```python
from build123d import *

# Parameters (mm, degrees)
CROQUIS1_W                   = 56
CROQUIS1_H                   = 82
CROQUIS1_W_2                 = 50
CROQUIS1_H_2                 = 76
EXTRUIR_L_MINA1_DEPTH        = 22
REDONDEO1_R                  = 4
REDONDEO2_R                  = 4
REDONDEO3_R                  = 4
REDONDEO4_R                  = 4
SALIENTE_EXTRUIR1_DEPTH      = 1
SALIENTE_EXTRUIR1_DEPTH_BACK = 1
REDONDEO5_R                  = 2
CROQUIS3_W                   = 6
CROQUIS3_H                   = 6.3
SALIENTE_EXTRUIR2_DEPTH      = 15.8
CROQUIS4_R                   = 0.75
CORTAR_EXTRUIR1_DEPTH        = 10
CROQUIS5_W                   = 10
CROQUIS5_H                   = 60.4
CORTAR_EXTRUIR2_DEPTH        = 10
CROQUIS6_W                   = 9
CROQUIS6_H                   = 67
CORTAR_EXTRUIR4_DEPTH        = 10
CROQUIS7_W                   = 3.2
CROQUIS7_H                   = 17
CORTAR_EXTRUIR5_DEPTH        = 10
CROQUIS8_W                   = 7.469429576
CROQUIS8_H                   = 3.762632311
SALIENTE_EXTRUIR3_DEPTH      = 22
CORTAR_EXTRUIR6_DEPTH        = 85
CROQUIS10_R                  = 1.25
CORTAR_EXTRUIR7_DEPTH        = 10
CROQUIS11_R                  = 1.1
CORTAR_EXTRUIR8_DEPTH        = 10


with BuildPart() as part:
    # Croquis1 → Extruir-Lámina1 (new body)
    with BuildSketch(Plane.XY):
        Rectangle(CROQUIS1_W, CROQUIS1_H)
        Rectangle(CROQUIS1_W_2, CROQUIS1_H_2, mode=Mode.SUBTRACT)
    extrude(amount=EXTRUIR_L_MINA1_DEPTH)

    # Redondeo1
    redondeo1_edges = [part.edges().sort_by_distance(p)[0] for p in [
        (-28, 41, 11),
    ]]
    fillet(redondeo1_edges, radius=REDONDEO1_R)

    # Redondeo2
    redondeo2_edges = [part.edges().sort_by_distance(p)[0] for p in [
        (28, 41, 11),
    ]]
    fillet(redondeo2_edges, radius=REDONDEO2_R)

    # Redondeo3
    redondeo3_edges = [part.edges().sort_by_distance(p)[0] for p in [
        (28, -41, 11),
    ]]
    fillet(redondeo3_edges, radius=REDONDEO3_R)

    # Redondeo4
    redondeo4_edges = [part.edges().sort_by_distance(p)[0] for p in [
        (-28, -41, 11),
    ]]
    fillet(redondeo4_edges, radius=REDONDEO4_R)

    # Croquis2 → Saliente-Extruir1 (add, two sides: drawn at the far end of the back side and taken through both)
    with BuildSketch(Plane.XY.offset(22).offset(-SALIENTE_EXTRUIR1_DEPTH_BACK)):
        with BuildLine():
            Line((-28, 37), (-28, -37))
            ThreePointArc((-28, -37), (-26.828427125, -39.828427125), (-24, -41))
            Line((-24, -41), (24, -41))
            ThreePointArc((24, -41), (26.828427125, -39.828427125), (28, -37))
            Line((28, -37), (28, 37))
            ThreePointArc((28, 37), (26.828427125, 39.828427125), (24, 41))
            Line((24, 41), (-24, 41))
            ThreePointArc((-24, 41), (-26.828427125, 39.828427125), (-28, 37))
        make_face()
    extrude(amount=SALIENTE_EXTRUIR1_DEPTH + SALIENTE_EXTRUIR1_DEPTH_BACK)

    # Redondeo5
    redondeo5_edges = [part.edges().sort_by_distance(p)[0] for p in [
        (-26.828427125, 39.828427125, 23),
        (-28, 0, 23),
        (-26.828427125, -39.828427125, 23),
        (0, -41, 23),
        (26.828427125, -39.828427125, 23),
        (28, 0, 23),
        (26.828427125, 39.828427125, 23),
        (0, 41, 23),
    ]]
    fillet(redondeo5_edges, radius=REDONDEO5_R)

    # Croquis3 → Saliente-Extruir2 (add)
    with BuildSketch(Plane(origin=(0, 0, 21), x_dir=(-1, 0, 0), z_dir=(0, 0, -1))):
        with Locations((-22, 34.85)):
            Rectangle(CROQUIS3_W, CROQUIS3_H)
        with Locations((-22, -34.85)):
            Rectangle(CROQUIS3_W, CROQUIS3_H)
        with Locations((22, 34.85)):
            Rectangle(CROQUIS3_W, CROQUIS3_H)
        with Locations((22, -34.85)):
            Rectangle(CROQUIS3_W, CROQUIS3_H)
    extrude(amount=SALIENTE_EXTRUIR2_DEPTH)

    # Croquis4 → Cortar-Extruir1 (cut)
    with BuildSketch(Plane(origin=(0, 0, 5.2), x_dir=(-1, 0, 0), z_dir=(0, 0, -1))):
        with Locations((-22, 34.5)):
            Circle(CROQUIS4_R)
        with Locations((22, 34.5)):
            Circle(CROQUIS4_R)
        with Locations((22, -34.5)):
            Circle(CROQUIS4_R)
        with Locations((-22, -34.5)):
            Circle(CROQUIS4_R)
    extrude(amount=-CORTAR_EXTRUIR1_DEPTH, mode=Mode.SUBTRACT)

    # Croquis5 → Cortar-Extruir2 (cut)
    with BuildSketch(Plane(origin=(0, 0, 21), x_dir=(-1, 0, 0), z_dir=(0, 0, -1))):
        with Locations((-20, 0)):
            Rectangle(CROQUIS5_W, CROQUIS5_H)
    extrude(amount=-CORTAR_EXTRUIR2_DEPTH, mode=Mode.SUBTRACT)

    # Croquis6 → Cortar-Extruir4 (cut)
    with BuildSketch(Plane(origin=(28, 0, 0), x_dir=(0, 0, -1), z_dir=(1, 0, 0))):
        with Locations((-11, 0)):
            Rectangle(CROQUIS6_W, CROQUIS6_H)
    extrude(amount=-CORTAR_EXTRUIR4_DEPTH, mode=Mode.SUBTRACT)

    # Croquis7 → Cortar-Extruir5 (cut)
    with BuildSketch(Plane(origin=(0, 0, 0), x_dir=(-1, 0, 0), z_dir=(0, 0, -1))):
        with Locations((25.4, -14.5)):
            Rectangle(CROQUIS7_W, CROQUIS7_H)
    extrude(amount=-CORTAR_EXTRUIR5_DEPTH, mode=Mode.SUBTRACT)

    # Croquis8 → Saliente-Extruir3 (add)
    with BuildSketch(Plane(origin=(0, 0, 0), x_dir=(-1, 0, 0), z_dir=(0, 0, -1))):
        with Locations((18.80938175, 42.881316156)):
            Rectangle(CROQUIS8_W, CROQUIS8_H)
        with Locations((-18.80938175, 42.881316156)):
            Rectangle(CROQUIS8_W, CROQUIS8_H)
        with Locations((-18.80938175, -42.881316156)):
            Rectangle(CROQUIS8_W, CROQUIS8_H)
        with Locations((18.80938175, -42.881316156)):
            Rectangle(CROQUIS8_W, CROQUIS8_H)
    extrude(amount=-SALIENTE_EXTRUIR3_DEPTH)

    # Croquis9 → Cortar-Extruir6 (cut)
    with BuildSketch(Plane(origin=(28, 0, 0), x_dir=(0, 0, -1), z_dir=(1, 0, 0))):
        Polygon((-21, 41), (0, 44.762632311), (0.10305202, 48.489025058), (-25.204298305, 46.436230698), (-22.314872849, 40.902663886), align=None)
        Polygon((-22.314872849, -40.902663886), (-21, -41), (0, -44.762632311), (0.10305202, -48.489025058), (-25.204298305, -46.436230698), align=None)
    extrude(amount=-CORTAR_EXTRUIR6_DEPTH, mode=Mode.SUBTRACT)

    # Croquis10 → Cortar-Extruir7 (cut)
    with BuildSketch(Plane(origin=(0, 0, 0), x_dir=(-1, 0, 0), z_dir=(0, 0, -1))):
        with Locations((-19, 41.25)):
            Circle(CROQUIS10_R)
        with Locations((19, 41.25)):
            Circle(CROQUIS10_R)
        with Locations((-19, -41.25)):
            Circle(CROQUIS10_R)
        with Locations((19, -41.25)):
            Circle(CROQUIS10_R)
    extrude(amount=-CORTAR_EXTRUIR7_DEPTH, mode=Mode.SUBTRACT)

    # Croquis11 → Cortar-Extruir8 (cut)
    with BuildSketch(Plane(origin=(0, 0, 5.2), x_dir=(-1, 0, 0), z_dir=(0, 0, -1))):
        with Locations((-22, 34.5)):
            Circle(CROQUIS11_R)
        with Locations((22, 34.5)):
            Circle(CROQUIS11_R)
        with Locations((22, -34.5)):
            Circle(CROQUIS11_R)
        with Locations((-22, -34.5)):
            Circle(CROQUIS11_R)
    extrude(amount=-CORTAR_EXTRUIR8_DEPTH, mode=Mode.SUBTRACT)


solid = part.part
```
Could you check a few things on this model? Use its own coordinates, in mm. A direction names the side the tool comes from. Round coordinates to 2 decimals unless told otherwise and drop trailing zeros. Loops run counter-clockwise (first coordinate to the right, second up) from the corner with the lowest first, then second, coordinate; pieces in that order, holes last. Notation, with made-up numbers: M 59,44 L 108,44 A23 ccw 108,78 Z; hole C 8,17 d11. An arc over 180 degrees is marked long. Write item = value, one per line.
1. I need wall thicknesses on probe 1 along Y at (x, z) = (11, 1.25); probe 2 along Y at (x, z) = (-22, 9.5); probe 3 along X at (y, z) = (24, 2). Which ranges of each line are inside material? Lowest first, please.
Results below:
probe_1 = -41 to -38, 38 to 41
probe_2 = -43.06 to -35.6, -33.4 to -31.7, 31.7 to 33.4, 35.6 to 43.06
probe_3 = -28 to -25, 25 to 28
2. Will these pins go through, and if not, where does the flat tip stop? P1, Ø1.1, axis at x = -22.5, y = -35, coming from the -Z side; P2, Ø1.6, axis at x = 23, z = 7.5, coming from the +Y side; P3, Ø1.9, axis at y = -43.5, z = 10.5, coming from the +X side.
Results below:
P1 = 5.2
P2 = 43.54
P3 = 22.54
3. I want a section at C-C, the plane z = 13.25. Count the separate pieces of the cut face and the enclosed holes in it, and give its area (3 significant figures).
Results below:
separate_pieces = 1
enclosed_holes = 2
area = 733 mm²
4. Which directions (+Z, -Z, +X, -X, +Y, -Y) give clear straight access to the entire face, cutting with the end or side of a thin tool? Please do faces 1 (the face through (15.075, 42, 8)), 2 (the face through (19, -41, 10)), 3 (the face through (22.544, 42, 8)).
Results below:
face_1 = +Z, -Z, +Y
face_2 = -Z
face_3 = +Z, -Z, +X, +Y
5. Thinking about a two-plate mould opening in Y: for faces 4 (the face through (-26.797, -39.859, 10.647)), 5 (the face through (20, -30.2, 22)), 6 (the face through (22.544, -42, 6)), which applies, +Y half, -Y half, draft (parallel to the pull), parting line (faces both ways), or undercut?
Results below:
face_4 = -Y half
face_5 = undercut
face_6 = draft
6. I want a section at B-B, the plane y = 34.5. Write out the boundary of the cut face in (x, z).
Results below:
outline = M -28,0 L -25,0 L -25,5.2 L -23.1,5.2 L -23.1,15.2 L -20.9,15.2 L -20.9,5.2 L -19,5.2 L -19,21 L 19,21 L 19,5.2 L 20.9,5.2 L 20.9,15.2 L 23.1,15.2 L 23.1,5.2 L 25,5.2 L 25,0 L 28,0 L 28,21 A2 ccw 26,23 L -26,23 A2 ccw -28,21 Z
7. I want a section at A-A, the plane x = -11.5. Write out the boundary of the cut face in (y, z).
Results below:
outline = M -41,0 L -38,0 L -38,21 L 38,21 L 38,0 L 41,0 L 41,21 L 40.98,21.29 A2 ccw 39,23 L -39,23 A2 ccw -40.98,21.29 L -41,21 Z
